```python
from build123d import *

# Parameters (mm, degrees)
SKETCH_W     = 86
SKETCH_H     = 74
SKETCH_R     = 3
PAD_DEPTH    = 2
SKETCH001_W  = 7
SKETCH001_H  = 12
PAD001_DEPTH = 9
SKETCH002_W  = 18.5
SKETCH002_H  = 35
PAD002_DEPTH = 14.5
SKETCH003_W  = 18.5
SKETCH003_H  = 0.2
PAD003_DEPTH = 6
SKETCH004_W  = 18.5
SKETCH004_H  = 6
PAD004_DEPTH = 23
SKETCH005_W  = 10
SKETCH005_H  = 20
PAD005_DEPTH = 16
SKETCH006_W  = 10
SKETCH006_H  = 10
PAD006_DEPTH = 7


with BuildPart() as part:
    # Sketch → Pad (new body)
    with BuildSketch(Plane.XY):
        Rectangle(SKETCH_W, SKETCH_H)
        with Locations((-38.5, 32.5)):
            Circle(SKETCH_R, mode=Mode.SUBTRACT)
        with Locations((38.5, 32.5)):
            Circle(SKETCH_R, mode=Mode.SUBTRACT)
        with Locations((-12.5, -29.5)):
            Circle(SKETCH_R, mode=Mode.SUBTRACT)
    extrude(amount=PAD_DEPTH)

    # Sketch001 → Pad001 (new body)
    with BuildSketch(Plane.XY.offset(2)):
        with Locations((-38, 22.5)):
            Rectangle(SKETCH001_W, SKETCH001_H)
        with Locations((-38, -1.5)):
            Rectangle(SKETCH001_W, SKETCH001_H)
        with Locations((-38, -25.5)):
            Rectangle(SKETCH001_W, SKETCH001_H)
    pad001 = extrude(amount=PAD001_DEPTH)

    # Mirrored: Pad001 across Sketch001 V_Axis
    add(pad001.mirror(Plane(origin=(0, 0, 2), x_dir=(0, 0, 1), z_dir=(1, 0, 0))))

    # Sketch002 → Pad002 (new body)
    with BuildSketch(Plane.XY.offset(2)):
        with Locations((-0.75, -2)):
            Rectangle(SKETCH002_W, SKETCH002_H)
    extrude(amount=PAD002_DEPTH)

    # Sketch003 → Pad003 (new body)
    with BuildSketch(Plane.XY.offset(16.5)):
        with Locations((-0.75, -19.4)):
            Rectangle(SKETCH003_W, SKETCH003_H)
    extrude(amount=PAD003_DEPTH)

    # Sketch004 → Pad004 (new body)
    with BuildSketch(Plane.XZ.offset(19.5)):
        with Locations((-0.75, 19.5)):
            Rectangle(SKETCH004_W, SKETCH004_H)
    extrude(amount=PAD004_DEPTH)

    # Sketch005 → Pad005 (new body)
    with BuildSketch(Plane.XY.offset(2)):
        with Locations((-27, 23.5)):
            Rectangle(SKETCH005_W, SKETCH005_H)
        with Locations((-27, 0.5)):
            Rectangle(SKETCH005_W, SKETCH005_H)
        with Locations((-27, -22.5)):
            Rectangle(SKETCH005_W, SKETCH005_H)
    pad005 = extrude(amount=PAD005_DEPTH)

    # Mirrored001: Pad005 across Sketch005 V_Axis
    add(pad005.mirror(Plane(origin=(0, 0, 2), x_dir=(0, 0, 1), z_dir=(1, 0, 0))))

    # Sketch006 → Pad006 (new body)
    with BuildSketch(Plane.XY.offset(2)):
        with Locations((-1, -36)):
            Rectangle(SKETCH006_W, SKETCH006_H)
    extrude(amount=PAD006_DEPTH)


solid = part.part
```
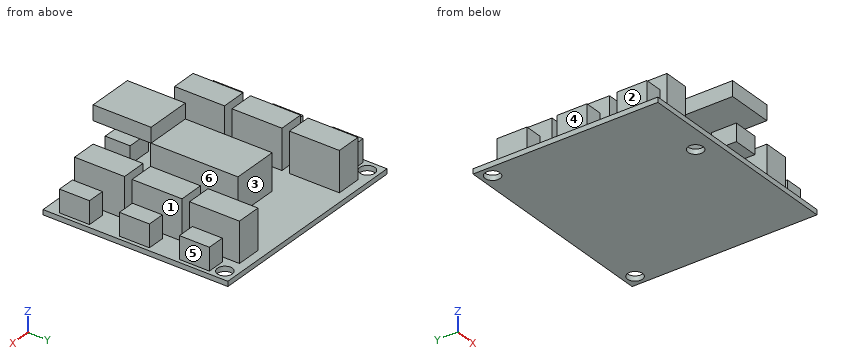
For this review, take the finished solid that the model builds, in its own axes (mm). Face numbers are marked on the shaded views. A direction names the side the tool comes from. Coordinates: 2 decimals unless noted, no trailing zeros. Loops run counter-clockwise (first coordinate to the right, second up) from the corner with the lowest first, then second, coordinate; pieces in that order, holes last. Notation, with made-up numbers: (-37.5, 68) - (-8.5, 68) arc R23 ccw to (-8.5, 95) - close; hole circle Ø2 at (73.25, -22). An arc over 180 degrees is marked (long way). Use one line per item in the form item = value. Start each with the question number.
1) Take a section at A-A (y = -29.5). State the section outline as (x, z) points, plus the area to 3 significant figures.
2) To check wall thickness, follow probe 1 along X at (y, z) = (-18, 6.25); probe 2 along X at (y, z) = (0.5, 3); probe 3 along Y at (x, z) = (38.5, 1.05). State the ranges of each line that lie inside material, in increasing order. Write a range as from..to.
3) Take a section at B-B (x = -12.5). State the section outline as (y, z) points.
4) Draft analysis for pull direction X (two halves, no side actions). For the marked faces 4, 5 and 6, state which applies: released by +X, released by -X, zero draft, split by the parting line, or undercut.
5) For the marked faces 1, 2 and 3, list the 3-axis set-ups (+Z, -Z, +X, -X, +Y, -Y) from which the entire face can be reached by the end or side of a thin tool; tool diameter is ignored.
6) For pin 1 (3 mm diameter, centred on x = 27.5, y = 2, fed in from +Z); pin 2 (13 mm diameter, centred on y = 0, z = 10, fed in from +X); pin 3 (10 mm diameter, centred on x = -6, y = 28.5, fed in from +Z), all flat-tipped, find the tip position at first contact; note any pin that passes through.
7) Take a section at D-D (y = -1). State the section outline as (x, z) points, plus the area to 3 significant figures.
8) Take a section at C-C (x = 0). State the section outline as (y, z) points, plus the area to 3 significant figures.
From the geometry:
q1.outline = (-43, 0) - (-15.5, 0) - (-15.5, 2) - (-22, 2) - (-22, 18) - (-32, 18) - (-32, 2) - (-34.5, 2) - (-34.5, 11) - (-41.5, 11) - (-41.5, 2) - (-43, 2) - close; (-10, 16.5) - (8.5, 16.5) - (8.5, 22.5) - (-10, 22.5) - close; (-9.5, 0) - (43, 0) - (43, 2) - (41.5, 2) - (41.5, 11) - (34.5, 11) - (34.5, 2) - (32, 2) - (32, 18) - (22, 18) - (22, 2) - (-9.5, 2) - close
q1.area = 717 mm2
q2.probe_1 = -32..-22, -10..8.5, 22..32
q2.probe_2 = -41.5..-34.5, -32..-22, -10..8.5, 22..32, 34.5..41.5
q2.probe_3 = -37..29.5, 35.5..37
q3.outline = (-37, 0) - (-32.5, 0) - (-32.5, 2) - (-37, 2) - close; (-26.5, 0) - (37, 0) - (37, 2) - (-26.5, 2) - close
q4.face_4 = released by -X
q4.face_5 = released by +X
q4.face_6 = undercut
q5.face_1 = +Z, +Y, -Y
q5.face_2 = +Z, -X, +Y, -Y
q5.face_3 = +Z, +Y
q6.pin_1 = 18
q6.pin_2 = 41.5
q6.pin_3 = 2
q7.outline = (-43, 0) - (43, 0) - (43, 2) - (41.5, 2) - (41.5, 11) - (34.5, 11) - (34.5, 2) - (32, 2) - (32, 18) - (22, 18) - (22, 2) - (8.5, 2) - (8.5, 16.5) - (-10, 16.5) - (-10, 2) - (-22, 2) - (-22, 18) - (-32, 18) - (-32, 2) - (-34.5, 2) - (-34.5, 11) - (-41.5, 11) - (-41.5, 2) - (-43, 2) - close
q7.area = 886 mm2
q8.outline = (-42.5, 16.5) - (-19.5, 16.5) - (-19.5, 2) - (-31, 2) - (-31, 9) - (-41, 9) - (-41, 2) - (-37, 2) - (-37, 0) - (37, 0) - (37, 2) - (15.5, 2) - (15.5, 16.5) - (-19.3, 16.5) - (-19.3, 22.5) - (-42.5, 22.5) - close
q8.area = 865 mm2
